Here's how the part is built. I have some questions about the finished solid (model axes, mm). Face numbers are marked on the shaded views. A direction names the side the tool comes from. Round coordinates to 2 decimals unless told otherwise and drop trailing zeros. Order: outer loops, then holes, each group sorted by start corner. A loop starts at its lowest first (then second) coordinate and runs counter-clockwise, first axis right, second up. Notation, with made-up numbers: (24, 55) - (74, 55) arc R31 ccw to (74, 94) - close; hole circle Ø8 at (6, 64.25). An arc over 180 degrees is marked (long way). One line per item, written item: value.
Autodesk Inventor part; units mm, degrees
ref_plane "YZ Plane" through (0, 0, 0) normal (1, 0, 0) x (0, 1, 0)
ref_plane "XZ Plane" through (0, 0, 0) normal (0, 1, 0) x (-1, 0, 0)
ref_plane "XY Plane" through (0, 0, 0) normal (0, 0, 1) x (1, 0, 0)
sketch "Sketch1" plane through (0, 0, 0) normal (0, 0, 1) x (1, 0, 0)
  line L0 (22.5, 44) -> (22.5, 25.6111)
  line L1 (13.5, 44) -> (13.5, 29.9618)
  arc A0 (22.5, 18.6538) -> (13.5, 23.9242) centre (0, -9.4487) ccw
  arc A1 (34.7379, 0) -> (22.5, 18.6538) centre (0, -9.4487) ccw
  arc A2 (40.5729, 0) -> (22.5, 25.6111) centre (0, -9.4487) ccw
  line L2 (13.5, 29.9618) -> (13.5, 23.9242)
  line L3 (13.5, 44) -> (22.5, 44)
  line L4 (34.7379, 0) -> (40.5729, 0)
  line L5 (0, -20.1384) -> (0, 54.6897)
  point P0 (0, 0)
revolve "Revolution1" add sketch "Sketch1" angle 360 about axis through (0, -10, 0) along (0, 1, 0)
sketch "Sketch2" plane through (0, 44, 0) normal (0, 1, 0) x (1, 0, 0)
  line L0 (-7, -13.5) -> (-7, -36)
  line L1 (-7, -36) -> (7, -36)
  line L2 (7, -36) -> (7, -13.5)
  line L3 (7, -13.5) -> (7, -11.5434)
  circle A0 centre (0, 0) radius 13.5
  line L4 (-7, -13.5) -> (-7, -11.5434)
  line L5 (-7, 13.5) -> (-7, 36)
  line L6 (-7, 36) -> (7, 36)
  line L7 (7, 36) -> (7, 13.5)
  line L8 (-7, 13.5) -> (-7, 11.5434)
  line L9 (7, 13.5) -> (7, 11.5434)
  dimension "d12" = 14
  dimension "d13" = 22.5
  dimension "d16" = 14
  dimension "d17" = 22.5
extrude "Extrusion1" add sketch "Sketch2" against normal blind 7.5 contours L4 A0 L3 L2 L1 L0 | L8 L5 L6 L7 L9 A0
sketch "Sketch3" plane through (-7, 44, -36) normal (0, 1, 0) x (1, 0, 0)
  circle A0 centre (7, -66.0778) radius 2.8
  circle A1 centre (7.0706, -5.9222) radius 2.8
  line L0 (14, -14.6166) -> (14, 0)
  point P0 (7, -36)
  dimension "d20" = 5.6
  dimension "d21" = 5.6
extrude "Extrusion2" cut sketch "Sketch3" against normal blind 7.5
properties part number "Vacuum Gripper"
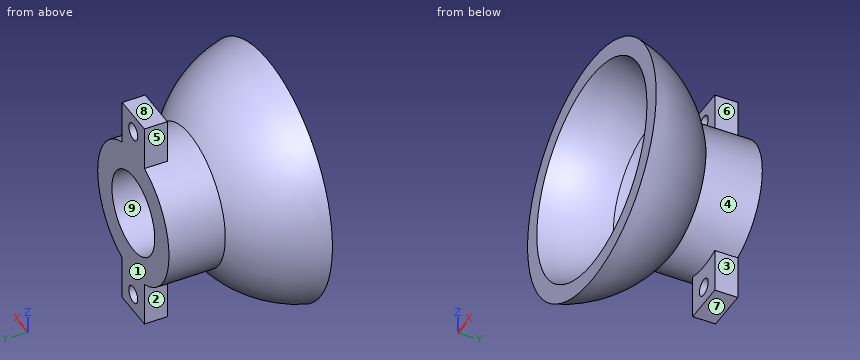
Q1. We'd pull the mould along Z, two halves only. Please class the marked faces 6, 7, 8 and 9: released by +Z, released by -Z, zero draft, split by the parting line, or undercut.
Results list:
face 6: zero draft
face 7: released by -Z
face 8: released by +Z
face 9: undercut
Q2. If we section it at A-A, the plane y = 35.5: Please give me the cut outline in (x, z).
Results list:
outline: circle Ø45 at (0, 0); hole circle Ø27 at (0, 0)
Q3. If we section it at B-B, the plane x = -1: Give the number of separate pieces and of enclosed holes in the cut face, then the cut area to 3 significant figures.
Results list:
separate pieces: 4
enclosed holes: 0
area: 840 mm²
Q4. If I drill on line 1 along Z through (x, y) = (0, 41); line 2 along Z through (x, y) = (0, 32), over which ranges is the centre line in solid material (lowest first)?
Results list:
line 1: -36 to -32.88, -27.28 to -13.5, 13.5 to 27.28, 32.88 to 36
line 2: -22.5 to -13.5, 13.5 to 22.5
Q5. Will these pins go through, and if not, where does the flat tip stop? pin 1 (4 mm diameter, centred on y = 21, z = 12, fed in from -X); pin 2 (10 mm diameter, centred on x = 8.5, y = 9, fed in from +Z); pin 3 (6.5 mm diameter, centred on x = 0.07, z = -30.08, fed in from -Y).
Results list:
pin 1: x = -28.13
pin 2: z = 38.74
pin 3: y = 4.16
Q6. Which directions (+Z, -Z, +X, -X, +Y, -Y) give clear straight access to the entire face, cutting with the end or side of a thin tool? Please do the marked faces 1, 2, 3, 4 and 5.
Results list:
face 1: +Z, -Z, +X, -X, +Y
face 2: -Z, -X, +Y
face 3: -Z, +X, +Y
face 4: none
face 5: +Z, -X, +Y
